from build123d import *

# Parameters (mm, degrees)
SKETCH_1_R          = 15
EXTRUDE_1_DEPTH     = 5
SHELL_1_T           = -1
CUT_EXTRUDE_1_DEPTH = 5
EXTRUDE_2_DEPTH     = 1
EXTRUDE_3_DEPTH     = 2.5
EXTRUDE_6_DEPTH     = 1
SKETCH_6_R          = 14
SKETCH_6_R_2        = 12.5
EXTRUDE_7_DEPTH     = 1.5


with BuildPart() as part:
    # 草图1 → 凸台-拉伸1 (new body)
    with BuildSketch(Plane(origin=(0, 0, 0), x_dir=(1, 0, 0), z_dir=(0, 1, 0))):
        with Locations(Location((0, 0, 0), (0, 0, 270))):
            Circle(SKETCH_1_R)
    extrude(amount=EXTRUDE_1_DEPTH)

    # 抽壳1
    shell_1_openings = [part.faces().sort_by_distance(p)[0] for p in [
        (0, 5, 0),
    ]]
    offset(amount=SHELL_1_T, openings=shell_1_openings, kind=Kind.INTERSECTION)

    # 草图2 → 切除-拉伸1 (cut)
    with BuildSketch(Plane(origin=(0, 1, 0), x_dir=(1, 0, 0), z_dir=(0, 1, 0))):
        with BuildLine():
            Line((-10.141362356, 4.260606713), (-9.848418855, -4.89986184))
            ThreePointArc((-9.848418855, -4.89986184), (-7.525588518, -8.022812316), (-4.260606713, -10.141362356))
            Line((-4.260606713, -10.141362356), (4.89986184, -9.848418855))
            ThreePointArc((4.89986184, -9.848418855), (8.022812316, -7.525588518), (10.141362356, -4.260606713))
            Line((10.141362356, -4.260606713), (9.848418855, 4.89986184))
            ThreePointArc((9.848418855, 4.89986184), (7.525588518, 8.022812316), (4.260606713, 10.141362356))
            Line((4.260606713, 10.141362356), (-4.89986184, 9.848418855))
            ThreePointArc((-4.89986184, 9.848418855), (-8.022812316, 7.525588518), (-10.141362356, 4.260606713))
        make_face()
    extrude(amount=-CUT_EXTRUDE_1_DEPTH, mode=Mode.SUBTRACT)

    # 草图3 → 凸台-拉伸2 (add)
    with BuildSketch(Plane(origin=(0, 3, 0), x_dir=(-1, 0, 0), z_dir=(0, -1, 0))):
        with BuildLine():
            Line((-14.790199458, 2.5), (-23.774977314, 2.5))
            Line((-23.774977314, 2.5), (-23.774977314, -2.5))
            Line((-23.774977314, -2.5), (-14.790199458, -2.5))
            ThreePointArc((-14.790199458, -2.5), (-15, 0), (-14.790199458, 2.5))
        make_face()
    extrude(amount=-EXTRUDE_2_DEPTH)

    # 草图4 → 凸台-拉伸3 (add, symmetric)
    with BuildSketch(Plane.XY):
        with BuildLine():
            Line((20.07401542, 13.910254038), (19.207990016, 13.410254038))
            Line((19.207990016, 13.410254038), (24.207990016, 4.75))
            ThreePointArc((24.207990016, 4.75), (24.207990016, 4.25), (23.774977314, 4))
            Line((23.774977314, 4), (23.774977314, 3))
            ThreePointArc((23.774977314, 3), (25.07401542, 3.75), (25.07401542, 5.25))
            Line((25.07401542, 5.25), (20.07401542, 13.910254038))
        make_face()
    extrude(amount=EXTRUDE_3_DEPTH, both=True)

    # 草图5 → 凸台-拉伸6 (add)
    with BuildSketch(Plane(origin=(21.07882825, 12.169867164, 0), x_dir=(0, 0, 1), z_dir=(-0.8660254037844399, -0.49999999999999806, 0))):
        with BuildLine():
            Line((6, 37.914379355), (-6, 37.914379355))
            Line((-6, 37.914379355), (-13.423393759, 25.056684201))
            ThreePointArc((-13.423393759, 25.056684201), (0, 1.806684201), (13.423393759, 25.056684201))
            Line((13.423393759, 25.056684201), (6, 37.914379355))
        make_face()
    extrude(amount=EXTRUDE_6_DEPTH)

    # 草图6 → 凸台-拉伸7 (add)
    with BuildSketch(Plane(origin=(20.212802846, 11.669867164, 0), x_dir=(0, 0, 1), z_dir=(-0.86602540378444, -0.4999999999999978, 0))):
        with Locations(Location((0, 17.306684201, 0), (0, 0, 90))):
            Circle(SKETCH_6_R)
        with Locations(Location((0, 17.306684201, 0), (0, 0, 270))):
            Circle(SKETCH_6_R_2, mode=Mode.SUBTRACT)
    extrude(amount=EXTRUDE_7_DEPTH)


solid = part.part
Model file for the job. Use its own axes, mm. A direction names the side the tool comes from. Give positions to 0.01 mm unless a question says otherwise; leave off trailing zeros. Order: outer loops, then holes, each group sorted by start corner. A loop starts at its lowest first (then second) coordinate and runs counter-clockwise, first axis right, second up. Notation, with made-up numbers: (73, 83) - (80, 83) arc R3 cw to (80, 88) - close; hole circle Ø1 at (-37, 2.25). An arc over 180 degrees is marked (long way). Write item = value, one per line. Start each with the question number.
1. Probe line 1 along Y through (x, z) = (6, 11); line 2 along X through (y, z) = (2.6, 0); line 3 along Y through (x, z) = (3, 10.5). List the from-to ranges inside material, lowest first.
2. Two-plate mould, pull along X, no slides. Class faces 1 (the flat face through (19, 4, 0)), 2 (the cylindrical face through (25.06, 3.73, 0.04)), 3 (the flat face through (4.86, 39.27, -9.66)): pulls with the +X half, pulls with the -X half, needs draft (parallel to the pull), parting line crosses it, or undercut.
3. Drop flat-ended pins along their axis: P1, Ø8, axis at x = -5.5, y = 11.5, coming from the -Z side; P2, Ø5.5, axis at x = 20.5, z = 0.5, coming from the +Y side; P3, Ø1, axis at x = 9, y = 4.5, coming from the -Z side; P4, Ø5, axis at y = 18.5, z = 4.5, coming from the +X side. Give the stop position or say it passes through.
4. Which spindle directions (+Z, -Z, +X, -X, +Y, -Y) get a long thin tool onto all of the face, cutting with end or side? Do faces 4 (the cylindrical face through (7.565, 0.507, -7.985)), 5 (the cylindrical face through (-13.67, 2.97, -3.03)), 6 (the flat face through (23.1, 7.3, -2.5)), 7 (the cylindrical face through (-7.565, 0.507, 7.985)), 8 (the flat face through (23.1, 7.3, 2.5)). Say none if no direction does.
5. Cut at A-A, the plane z = -9. List the corners of the cut face in (x, y).
6. Cut at D-D, the plane x = -8.5. List the corners of the cut face in (y, z), and give its area (3 significant figures).
7. Cut at C-C, the plane x = 0. List the corners of the cut face in (y, z), and give its area (3 significant figures).
8. Cut at B-B, the plane z = 1. List the corners of the cut face in (x, y), and give its area (3 significant figures).
Taken from the geometry:
q1.line_1 = 0 to 1, 33.29 to 33.45, 36.29 to 37.24
q1.line_2 = -15 to -14, 14 to 15
q1.line_3 = 0 to 1
q2.face_1 = undercut
q2.face_2 = pulls with the +X half
q2.face_3 = pulls with the -X half
q3.P1 = through
q3.P2 = 17.94
q3.P3 = -12.36
q3.P4 = 18.87
q4.face_4 = -Y
q4.face_5 = none
q4.face_6 = -Z, +X, -Y
q4.face_7 = +Y, -Y
q4.face_8 = +Z, +X, -Y
q5.outline = (-12, 0) - (-6.32, 0) - (-6.32, 1) - (-10.72, 1) - (-10.72, 5) - (-12, 5) - close; (3.85, 40) - (6.2, 35.94) - (4.9, 35.19) - (5.92, 33.42) - (7.22, 34.17) - (15.9, 19.15) - (14.6, 18.4) - (15.62, 16.62) - (16.92, 17.37) - (17.87, 15.73) - (18.74, 16.23) - (4.72, 40.5) - close; (6.32, 0) - (12, 0) - (12, 5) - (10.72, 5) - (10.72, 1) - (6.32, 1) - close
q6.outline = (0, -12.36) - (5, -12.36) - (5, -11.12) - (1, -11.12) - (1, -6.98) - (0, -6.98) - close; (0, 6.98) - (1, 6.98) - (1, 11.12) - (5, 11.12) - (5, 12.36) - (0, 12.36) - close
q6.area = 20.6 mm²
q7.outline = (0, -15) - (5, -15) - (5, -14) - (1, -14) - (1, -10.01) - (0, -10.01) - close; (0, 10.01) - (1, 10.01) - (1, 14) - (5, 14) - (5, 15) - (0, 15) - close
q7.area = 18.0 mm²
q8.outline = (-14.97, 0) - (-9.97, 0) - (-9.97, 1) - (-13.96, 1) - (-13.96, 5) - (-14.97, 5) - close; (1.26, 44.5) - (4.58, 38.75) - (3.28, 38) - (4.03, 36.7) - (5.33, 37.45) - (17.79, 15.87) - (16.49, 15.12) - (17.24, 13.81) - (18.54, 14.56) - (24.21, 4.75) arc R0.5 cw to (23.77, 4) - (14.97, 4) - (14.97, 5) - (13.96, 5) - (13.96, 1) - (10.04, 1) - (10.04, 0) - (14.97, 0) - (14.97, 3) - (23.77, 3) arc R1.5 ccw to (25.07, 5.25) - (2.12, 45) - close
q8.area = 79.3 mm²
